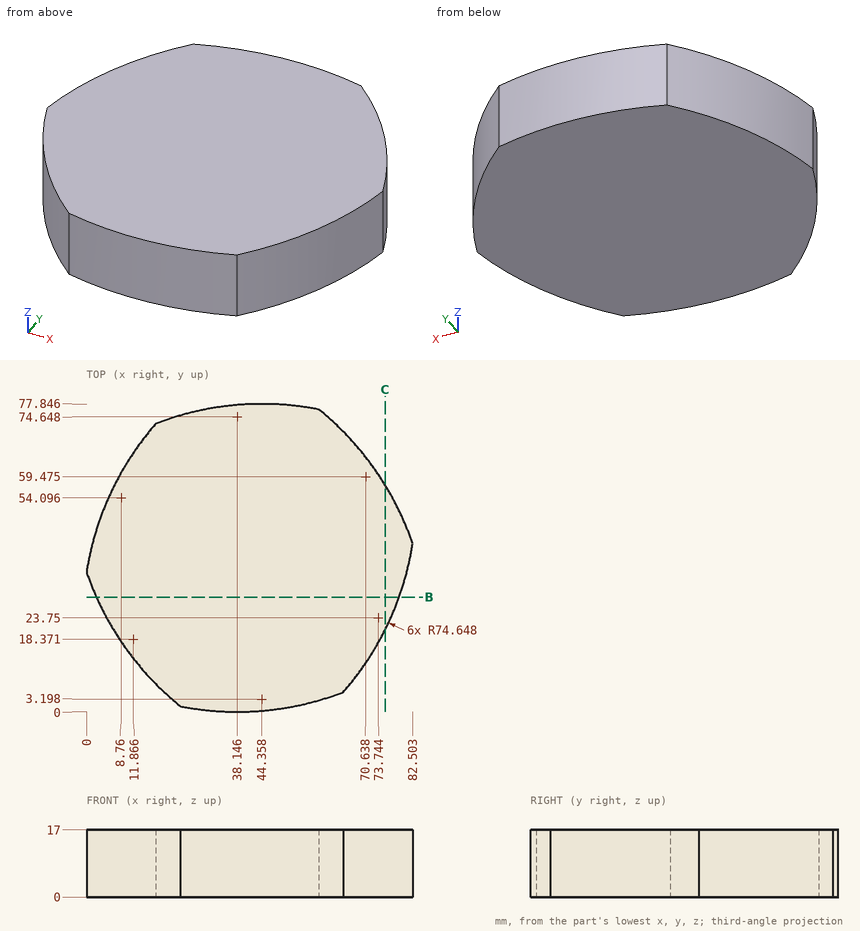
Source: three-view drawing plus pictorial views. Frame: mm from the lowest corner of the part. Round coordinates to 2 decimals unless told otherwise and drop trailing zeros. Loops run counter-clockwise (first coordinate to the right, second up) from the corner with the lowest first, then second, coordinate; pieces in that order, holes last. Notation, with made-up numbers: (-18, -14) - (5, -14) arc R20 ccw to (5, 5) - close; hole circle Ø10 at (-5.5, 31). An arc over 180 degrees is marked (long way). Write each question's results on one line, items separated by ' | '. Start each with the question number.
1) Line query: probe 1 along Y at (x, z) = (70, 13.5) (1 decimal); probe 2 along Y at (x, z) = (64, 6.75) (1 decimal); probe 3 along X at (y, z) = (72.5, 6). Output: solid intervals per line, ascending. Write a range as [from, to].
2) First-contact query: P1, Ø2, axis at x = 59, z = 3, coming from the +Y side; P2, Ø2, axis at y = 29.5, z = 3.5, coming from the -X side; P3, Ø8, axis at x = 71, z = 7, coming from the -Y side. Flat tips, straight axial feed; report the tip coordinate or a pass-through.
3) Cut plane B-B on y = 29. Return loops of the section in (x, z).
4) Cut plane C-C on x = 75.5. Return loops of the section in (y, z).
Verdict:
1) probe 1: y = [11.4, 65.2] | probe 2: y = [4.6, 71.8] | probe 3: x = [17.21, 63.27]
2) P1: stops at y = 76.59 | P2: stops at x = 1.84 | P3: stops at y = 7.4
3) outline: (2.49, 0) - (79.06, 0) - (79.06, 17) - (2.49, 17) - close
4) outline: (20.66, 0) - (57.4, 0) - (57.4, 17) - (20.66, 17) - close
